Here's how the part is built. I have some questions about the finished solid (model axes, mm). Give positions to 0.01 mm unless a question says otherwise; leave off trailing zeros. Write each loop counter-clockwise with the first axis right and the second up, starting at its lowest first coordinate (ties: lowest second). Pieces come first, ordered by that corner, then holes. Notation, with made-up numbers: (-34, 10) -> (18, 10) arc R26 cw to (18, 27) -> close; hole circle Ø7 at (-37, 84). An arc over 180 degrees is marked (long way). Answer as CSV lines item,"result". Start each with the question number.
from build123d import *

# Parameters (mm, degrees)
F0_R     = 3.25
F1_DEPTH = 12
F2_SIZE  = 3.25
F3_SIZE  = 0.5


with BuildPart() as f1:
    # F0 (on Right) → F1 (new body)
    with BuildSketch(Plane.YZ):
        Polygon((7.5, 20), (-71.5, 20), (-71.5, -20), (71.5, -20), (71.5, 20), (71.5, 40), (47.5, 40), align=None)
        with Locations((-61.5, -10)):
            Circle(F0_R, mode=Mode.SUBTRACT)
        with Locations((-31.5, -10)):
            Circle(F0_R, mode=Mode.SUBTRACT)
        with Locations((-1.5, -10)):
            Circle(F0_R, mode=Mode.SUBTRACT)
        with Locations((53.5, 5.999998)):
            Circle(F0_R, mode=Mode.SUBTRACT)
        with Locations((65.5, 5.999998)):
            Circle(F0_R, mode=Mode.SUBTRACT)
        with Locations((-61.5, 10)):
            Circle(F0_R, mode=Mode.SUBTRACT)
        with Locations((-31.5, 10)):
            Circle(F0_R, mode=Mode.SUBTRACT)
        with Locations((-1.5, 10)):
            Circle(F0_R, mode=Mode.SUBTRACT)
        with Locations((53.5, 33.999998)):
            Circle(F0_R, mode=Mode.SUBTRACT)
        with Locations((65.5, 33.999998)):
            Circle(F0_R, mode=Mode.SUBTRACT)
    extrude(amount=F1_DEPTH)

    # F2
    f2_edges = [f1.edges().sort_by_distance(p)[0] for p in [
        (12, -64.75, 10),
        (12, -34.75, 10),
        (12, -4.75, 10),
        (12, -4.75, -10),
        (12, -34.75, -10),
        (12, -64.75, -10),
    ]]
    chamfer(f2_edges, length=F2_SIZE)

    # F3
    f3_edges = [f1.edges().sort_by_distance(p)[0] for p in [
        (0, -4.75, -10),
        (0, -4.75, 10),
        (0, -34.75, 10),
        (0, -34.75, -10),
        (0, -64.75, -10),
        (0, -64.75, 10),
        (6, 68.75, 33.999998),
        (0, 62.25, 33.999998),
        (12, 62.25, 33.999998),
        (6, 56.75, 33.999998),
        (0, 50.25, 33.999998),
        (12, 50.25, 33.999998),
        (6, 56.75, 5.999998),
        (0, 50.25, 5.999998),
        (12, 50.25, 5.999998),
        (6, 68.75, 5.999998),
        (0, 62.25, 5.999998),
        (12, 62.25, 5.999998),
    ]]
    chamfer(f3_edges, length=F3_SIZE)


solid = f1.part
Item 1: We'd pull the mould along Z, two halves only. Please class faces 1 (the face through (8.95, -34.24, -12.1)), 2 (the face through (6, -1, -20)), 3 (the face through (12, 15, 4)), 4 (the face through (6, 60, 40)): released by +Z, released by -Z, zero draft, split by the parting line, or undercut.
Item 2: If we section it at B-B (z = -10): Please give me the cut outline in (x, y), and give its area (3 significant figures).
Item 3: If we section it at D-D (y = 53.5): Please give me the cut outline in (x, z), and give its area (3 significant figures).
Item 4: If I drill on line 1 (Z direction, x = 6.25, y = -31.5); line 2 (Z direction, x = 7.5, y = 53.5); line 3 (Y direction, x = 1.5, z = 8), over which ranges is the centre line in solid material (lowest first)? Write a range as [from, to].
Item 5: If we section it at A-A (y = -61.5): Please give me the cut outline in (x, z), and give its area (3 significant figures).
Item 6: I'm going to push flat-ended pins straight in: pin 1 (10.5 mm diameter, centred on y = -61.5, z = 10, fed in from +X); pin 2 (1 mm diameter, centred on x = 9, y = -55.5, fed in from +Z); pin 3 (10 mm diameter, centred on y = 5.5, z = -2.5, fed in from -X); pin 4 (5 mm diameter, centred on x = 2.5, z = 29, fed in from -Y). Where does each tip first touch, or does it pass through?
Item 7: If we section it at C-C (x = 3.75): State how many separate pieces and enclosed holes the cut face has, and give its area (3 significant figures).
Final values:
1,face 1,"undercut"
1,face 2,"released by -Z"
1,face 3,"zero draft"
1,face 4,"released by +Z"
2,outline,"(0, -71.5) -> (12, -71.5) -> (12, -68) -> (8.75, -64.75) -> (0.5, -64.75) -> (0, -65.25) -> close; (0, -57.75) -> (0.5, -58.25) -> (8.75, -58.25) -> (12, -55) -> (12, -38) -> (8.75, -34.75) -> (0.5, -34.75) -> (0, -35.25) -> close; (0, -27.75) -> (0.5, -28.25) -> (8.75, -28.25) -> (12, -25) -> (12, -8) -> (8.75, -4.75) -> (0.5, -4.75) -> (0, -5.25) -> close; (0, 2.25) -> (0.5, 1.75) -> (8.75, 1.75) -> (12, 5) -> (12, 71.5) -> (0, 71.5) -> close"
2,area,"1,450 mm2"
3,outline,"(0, -20) -> (12, -20) -> (12, 2.25) -> (11.5, 2.75) -> (0.5, 2.75) -> (0, 2.25) -> close; (0, 9.75) -> (0.5, 9.25) -> (11.5, 9.25) -> (12, 9.75) -> (12, 30.25) -> (11.5, 30.75) -> (0.5, 30.75) -> (0, 30.25) -> close; (0, 37.75) -> (0.5, 37.25) -> (11.5, 37.25) -> (12, 37.75) -> (12, 40) -> (0, 40) -> close"
3,area,"563 mm2"
4,line 1,"[-20, -13.25], [-6.75, 6.75], [13.25, 20]"
4,line 2,"[-20, 2.75], [9.25, 30.75], [37.25, 40]"
4,line 3,"[-71.5, -64.06], [-58.94, -34.06], [-28.94, -4.06], [1.06, 50.94], [56.06, 62.94], [68.06, 71.5]"
5,outline,"(0, -20) -> (12, -20) -> (12, -16.5) -> (8.75, -13.25) -> (0.5, -13.25) -> (0, -13.75) -> close; (0, -6.25) -> (0.5, -6.75) -> (8.75, -6.75) -> (12, -3.5) -> (12, 3.5) -> (8.75, 6.75) -> (0.5, 6.75) -> (0, 6.25) -> close; (0, 13.75) -> (0.5, 13.25) -> (8.75, 13.25) -> (12, 16.5) -> (12, 20) -> (0, 20) -> close"
5,area,"302 mm2"
6,pin 1,"x = 10.75"
6,pin 2,"z = 20"
6,pin 3,"x = 0"
6,pin 4,"y = 20.5"
7,separate pieces,"1"
7,enclosed holes,"10"
7,area,"6,270 mm2"
